For this review, take the finished solid that the model builds, in its own axes (mm). Face numbers are marked on the shaded views. A direction names the side the tool comes from. Round coordinates to 2 decimals unless told otherwise and drop trailing zeros. Write each loop counter-clockwise with the first axis right and the second up, starting at its lowest first coordinate (ties: lowest second). Pieces come first, ordered by that corner, then holes. Notation, with made-up numbers: (76, 9.5) - (100, 9.5) arc R5 ccw to (100, 16.5) - close; hole circle Ø8 at (70.25, 11). An arc over 180 degrees is marked (long way). Answer in a Markdown table with one row per item. Add a question column.
from build123d import *

# Parameters (mm, degrees)
SKIZZE1_W                       = 100
SKIZZE1_H                       = 100
AUFSATZ_LINEAR_AUSTRAGEN1_DEPTH = 50
SKIZZE2_OUTSIDE_W               = 132
SKIZZE2_OUTSIDE_H               = 82
SCHNITT_LINEAR_AUSTRAGEN1_DEPTH = 101
SKIZZE3_OUTSIDE_W               = 142.594
SKIZZE3_OUTSIDE_H               = 132
SKIZZE3_OUTSIDE_W_2             = 12
SKIZZE3_OUTSIDE_H_2             = 12
SCHNITT_LINEAR_AUSTRAGEN2_DEPTH = 58.357643635
SCHNITT_LINEAR_AUSTRAGEN3_DEPTH = 50


with BuildPart() as part:
    # Skizze1 → Aufsatz-Linear austragen1 (new body)
    with BuildSketch(Plane(origin=(0, 0, 0), x_dir=(1, 0, 0), z_dir=(0, 1, 0))):
        with Locations((50, 50)):
            Rectangle(SKIZZE1_W, SKIZZE1_H)
    extrude(amount=AUFSATZ_LINEAR_AUSTRAGEN1_DEPTH)

    # Skizze2 outside → Schnitt-Linear austragen1 (cut, through all)
    with BuildSketch(Plane.XY):
        with Locations((50, 25)):
            Rectangle(SKIZZE2_OUTSIDE_W, SKIZZE2_OUTSIDE_H)
        Polygon((0, 0), (0, 70.020753821), (100, 0), align=None, mode=Mode.SUBTRACT)
    extrude(amount=-SCHNITT_LINEAR_AUSTRAGEN1_DEPTH, mode=Mode.SUBTRACT)

    # Skizze3 outside → Schnitt-Linear austragen2 (cut, through all)
    with BuildSketch(Plane(origin=(32.898992834, 46.984631039, 0), x_dir=(0.819152044, -0.573576436, 0), z_dir=(0.573576436, 0.819152044, 0))):
        with Locations((26.618, 50)):
            Rectangle(SKIZZE3_OUTSIDE_W, SKIZZE3_OUTSIDE_H)
        Polygon((81.915204429, 37.859878609), (81.915204429, 55.30029111), (78.408084137, 65.614823426), (35.984131413, 65.614823426), (35.984131413, 51.664109902), (54.501889142, 42.446196436), (68.128544963, 42.446196436), (73.025747531, 37.859878609), align=None, mode=Mode.SUBTRACT)
        with Locations((65.828544963, 48.696196436)):
            Rectangle(SKIZZE3_OUTSIDE_W_2, SKIZZE3_OUTSIDE_H_2)
    extrude(amount=-SCHNITT_LINEAR_AUSTRAGEN2_DEPTH, mode=Mode.SUBTRACT)

    # Skizze4 → Schnitt-Linear austragen3 (cut)
    with BuildSketch(Plane(origin=(0, 0, 0), x_dir=(1, 0, 0), z_dir=(0, 1, 0))):
        Polygon((62.375467643, 65.614823426), (62.375467643, 51.664109902), (77.544326742, 42.446196436), (62.375467643, 16.747939689), (28.386649176, 16.747939689), (28.386649176, 99.890537097), (62.375467643, 99.890537097), align=None)
    extrude(amount=SCHNITT_LINEAR_AUSTRAGEN3_DEPTH, mode=Mode.SUBTRACT)


solid = part.part
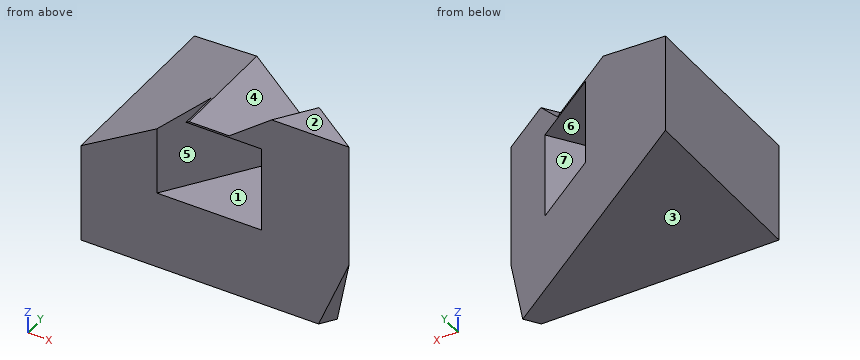
Q1. To check wall thickness, follow probe 1 along Z at (x, y) = (84, 10.5); probe 2 along X at (y, z) = (1.25, -46.5); probe 3 along X at (y, z) = (2.25, -54.5). State the ranges of each line that lie inside material, in increasing order.
Q2. Insertion check: pin 1 Ø14 at (x, y) = (79.5, 4.5) entering from +Z; pin 2 Ø1.5 at (x, z) = (85, -41) entering from +Y; pin 3 Ø8 at (y, z) = (16.5, -49.5) entering from +X; pin 4 Ø1.5 at (y, z) = (21.5, -44.5) entering from -X. Each pin has a flat end and moves straight along its axis. Give the tip position at first contact, or say it passes through.
Q3. Add section D-D on z = -62. State the section outline as (x, y) points.
Q4. Draft analysis for pull direction Z (two halves, no side actions). For the marked faces 1, 2 and 3, state which applies: released by +Z, released by -Z, zero draft, split by the parting line, or undercut.
Q5. Add section C-C on x = 69.5. State the section outline as (y, z) points.
Q6. Add section B-B on y = 1.5. State the section outline as (x, z) points.
Q7. Tool access review of the marked faces 4, 5, 6 and 7: name each direction out of +Z, -Z, +X, -X, +Y, -Y from which nothing blocks a thin tool from reaching the whole face with its end or side.
Q8. Add section A-A on z = -47.25. State the section outline as (x, y) points, then the cut area to 3 significant figures.
Answer sheet:
| question | item | result |
|---|---|---|
| 1 | probe 1 | z = -65.61 to -54.7, -42.7 to -42.45 |
| 1 | probe 2 | x = 70.87 to 73.91, 88.56 to 98.21 |
| 1 | probe 3 | x = 62.38 to 74.61, 89.26 to 96.79 |
| 2 | pin 1 | stops at z = -41.12 |
| 2 | pin 2 | stops at y = 1.68 |
| 2 | pin 3 | stops at x = 81.91 |
| 2 | pin 4 | passes through |
| 3 | outline | (62.38, 0) - (97.22, 0) - (98.13, 1.31) - (62.38, 26.34) - close |
| 4 | face 1 | undercut |
| 4 | face 2 | released by +Z |
| 4 | face 3 | released by -Z |
| 5 | outline | (0, -65.61) - (21.36, -65.61) - (21.36, -47.33) - (0, -47.33) - close |
| 6 | outline | (62.38, -65.61) - (96.77, -65.61) - (97.86, -62.99) - (97.86, -37.86) - (90.2, -37.86) - (84.22, -42.45) - (77.54, -42.45) - (77.13, -42.7) - (88.74, -42.7) - (88.74, -54.7) - (74.09, -54.7) - (74.09, -44.55) - (62.38, -51.66) - close |
| 7 | face 4 | +Z, -X, +Y |
| 7 | face 5 | -Y |
| 7 | face 6 | none |
| 7 | face 7 | +Y |
| 8 | outline | (69.64, 0) - (73.04, 0) - (81.91, 12.67) - (69.64, 21.26) - close; (87.69, 0) - (100, 0) - (91.74, 5.79) - close |
| 8 | area | 188 mm² |
